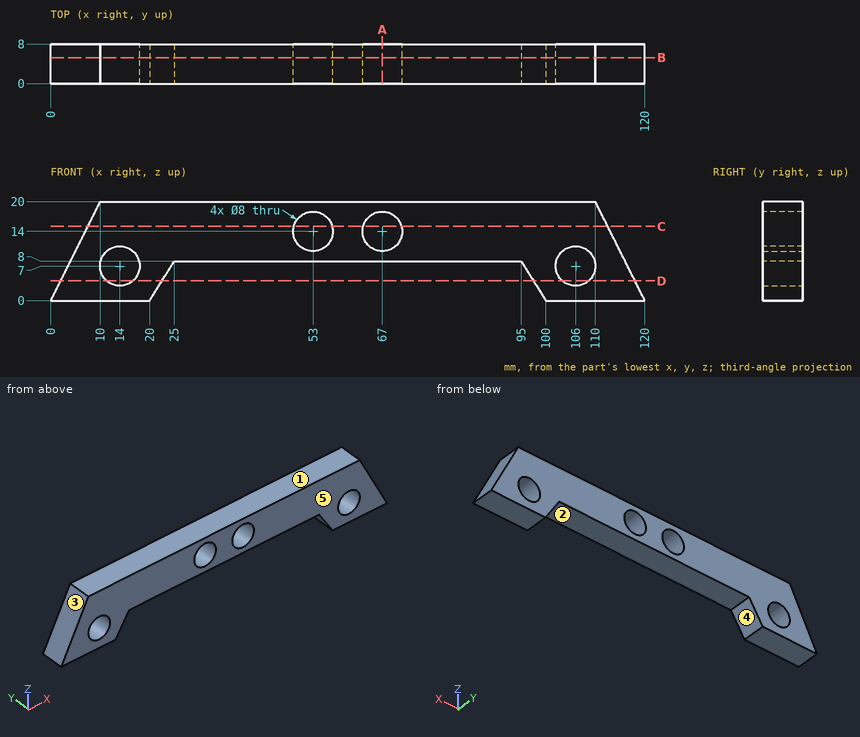
Source: three-view drawing plus pictorial views. Frame: mm from the lowest corner of the part. A direction names the side the tool comes from. Give positions to 0.01 mm unless a question says otherwise; leave off trailing zeros. Order: outer loops, then holes, each group sorted by start corner. A loop starts at its lowest first (then second) coordinate and runs counter-clockwise, first axis right, second up. Notation, with made-up numbers: M 14,58.25 L 39,58.25 A17 cw 39,75.25 Z; hole C 40.25,83 d11. An arc over 180 degrees is marked long. One line per question, with ' | ' between items. Start each with the question number.
1. Pull-direction query (X, two-part tool) for the marked faces 1, 2 and 3; classes: released by +X, released by -X, zero draft, split by the parting line, or undercut.
2. Section query B-B (y = 5.25). Return the cut outline in (x, z), and give its area (3 significant figures).
3. Section query C-C (z = 15). Return the cut outline in (x, y), and give its area (3 significant figures).
4. Material intervals for probe 1 along X at (y, z) = (6, 13.75) (3 decimals); probe 2 along X at (y, z) = (1.5, 5) (3 decimals); probe 3 along X at (y, z) = (6, 14), sorted ascending. Write a range as [from, to].
5. First-contact query: pin 1 Ø3 at (y, z) = (1, 5) entering from -X; pin 2 Ø2 at (x, y) = (92, 5) entering from -Z; pin 3 Ø5 at (x, z) = (53, 14) entering from +Y; pin 4 Ø4 at (y, z) = (4, 14.5) entering from -X. Flat tips, straight axial feed; report the tip coordinate or a pass-through.
6. Section query D-D (z = 4). Return the cut outline in (x, y).
7. Section query A-A (x = 67). Return the cut outline in (y, z), and give its area (3 significant figures).
8. Access query for the marked faces 4 and 5. Directions: +Z, -Z, +X, -X, +Y, -Y. A direction counts if a zero-diameter tool reaches every point of the face in a straight line with its end or side. Return the directions, or none.
Here are the results:
1) face 1: zero draft | face 2: undercut | face 3: released by -X
2) outline: M 0,0 L 20,0 L 25,8 L 95,8 L 100,0 L 120,0 L 110,20 L 10,20 Z; hole C 14,7 d8; hole C 53,14 d8; hole C 67,14 d8; hole C 106,7 d8 | area: 1,400 mm²
3) outline: M 7.5,0 L 49.13,0 L 49.13,8 L 7.5,8 Z; M 56.87,0 L 63.13,0 L 63.13,8 L 56.87,8 Z; M 70.87,0 L 112.5,0 L 112.5,8 L 70.87,8 Z | area: 716 mm²
4) probe 1: [6.875, 49.008], [56.992, 63.008], [70.992, 113.125] | probe 2: [2.5, 10.536], [17.464, 23.125], [96.875, 102.536], [109.464, 117.5] | probe 3: [7, 49], [57, 63], [71, 113]
5) pin 1: x = 1.75 | pin 2: z = 8 | pin 3: through | pin 4: x = 6.25
6) outline: M 2,0 L 11.35,0 L 11.35,8 L 2,8 Z; M 16.65,0 L 22.5,0 L 22.5,8 L 16.65,8 Z; M 97.5,0 L 103.35,0 L 103.35,8 L 97.5,8 Z; M 108.65,0 L 118,0 L 118,8 L 108.65,8 Z
7) outline: M 0,8 L 8,8 L 8,10 L 0,10 Z; M 0,18 L 8,18 L 8,20 L 0,20 Z | area: 32.0 mm²
8) face 4: -Z, +Y, -Y | face 5: +Z, -Z, +X, -X, -Y
